```python
from build123d import *

# Parameters (mm, degrees)
SKETCH007_R     = 6
PAD006_DEPTH    = 30
POCKET_DEPTH    = 27
SKETCH009_W     = 9
SKETCH009_H     = 11
SKETCH009_H_2   = 3
POCKET001_DEPTH = 2


with BuildPart() as part:
    # Sketch007 → Pad006 (new body)
    with BuildSketch(Plane.XY):
        with BuildLine():
            ThreePointArc((83.613695, 29), (-88.5, 0), (83.613695, -29))
            Line((88.613695, -29), (83.613695, -29))
            Line((88.613695, 29), (88.613695, -29))
            Line((83.613695, 29), (88.613695, 29))
        make_face()
        with Locations((43.046276, 63.61895)):
            Circle(SKETCH007_R, mode=Mode.SUBTRACT)
        with Locations((54.046276, 52)):
            Circle(SKETCH007_R, mode=Mode.SUBTRACT)
        with Locations((65.046276, 40.38105)):
            Circle(SKETCH007_R, mode=Mode.SUBTRACT)
    extrude(amount=-PAD006_DEPTH)

    # Sketch008 → Pocket (cut)
    with BuildSketch(Plane.XY):
        with BuildLine():
            ThreePointArc((83.230103, 27), (-87.5, 0), (83.230103, -27))
            Line((83.230103, -27), (87.230103, -27))
            Line((87.230103, -27), (87.230103, 27))
            Line((87.230103, 27), (83.230103, 27))
        make_face()
    extrude(amount=-POCKET_DEPTH, mode=Mode.SUBTRACT)

    # Sketch009 (on Face6 of Pocket) → Pocket001 (cut)
    with BuildSketch(Plane.YZ.offset(88.613695)):
        with Locations((18, -19.5)):
            Rectangle(SKETCH009_W, SKETCH009_H)
        with Locations((-13.5, -23.5)):
            Rectangle(SKETCH009_W, SKETCH009_H_2)
    extrude(amount=-POCKET001_DEPTH, mode=Mode.SUBTRACT)


solid = part.part
```
CAD build for the part. Positions are in the model's coordinates, mm. A direction names the side the tool comes from. Coordinates: 2 decimals unless noted, no trailing zeros. Loops run counter-clockwise (first coordinate to the right, second up) from the corner with the lowest first, then second, coordinate; pieces in that order, holes last. Notation, with made-up numbers: (38.5, 88) - (89.5, 88) arc R28 ccw to (89.5, 125) - close; hole circle Ø10 at (-24.75, 43). An arc over 180 degrees is marked (long way). Return JSON: item names as keys, results as strings.
1. Mould opens along X. For faces 1 (the cylindrical face through (46.27, 68.68, -28.48)), 2 (the flat face through (85, -27, -13)), 3 (the flat face through (86, 29, -15)), 4 (the cylindrical face through (-88.43, 3.48, -14.79)) say: released by +X, released by -X, zero draft, split by the parting line, or undercut.
Result:
{"face 1": "undercut", "face 2": "undercut", "face 3": "zero draft", "face 4": "split by the parting line"}
2. Band-saw the part on D-D (x = 0). Give the cut face in (y, z), and give its area (3 significant figures).
Result:
{"outline": "(-88.5, -30) - (88.5, -30) - (88.5, 0) - (87.5, 0) - (87.5, -27) - (-87.5, -27) - (-87.5, 0) - (-88.5, 0) - close", "area": "585 mm2"}
3. Band-saw the part on A-A (z = -11.75). Give the cut face in (x, y).
Result:
{"outline": "(83.61, -29) - (88.61, -29) - (88.61, 29) - (83.61, 29) arc R88.5 ccw (long way) to start; hole (83.23, -27) - (87.23, -27) - (87.23, 27) - (83.23, 27) arc R87.5 ccw (long way) to start"}
4. Band-saw the part on B-B (x = 43). Give the cut face in (y, z).
Result:
{"outline": "(-77.35, -30) - (57.62, -30) - (57.62, -27) - (-76.21, -27) - (-76.21, 0) - (-77.35, 0) - close; (69.62, -30) - (77.35, -30) - (77.35, 0) - (76.21, 0) - (76.21, -27) - (69.62, -27) - close"}
5. Band-saw the part on C-C (y = -13.5). Give the cut face in (x, z), and give its area (3 significant figures).
Result:
{"outline": "(-87.46, -30) - (88.61, -30) - (88.61, -25) - (87.23, -25) - (87.23, -27) - (-86.45, -27) - (-86.45, 0) - (-87.46, 0) - close; (87.23, -22) - (88.61, -22) - (88.61, 0) - (87.23, 0) - close", "area": "589 mm2"}
6. Probe L1, parallel to Y at x = 0, z = -19.75; L2, parallel to Z at x = -25.5, y = -29; L3, parallel to X at y = 36.5, z = -4.5. List the from-to ranges inside material, lowest first. Write a range as from..to.
Result:
{"L1": "y = -88.5..-87.5, 87.5..88.5", "L2": "z = -30..-27", "L3": "x = -80.62..-79.52, 79.52..80.62"}
7. 3-axis set-ups, long thin cutter, end or side, ignore diameter. For faces 5 (the flat face through (86, -29, -15)), 6 (the cylindrical face through (60.285, 36.73, -28.479)), 7 (the flat face through (-1, 1, -27)): which of +Z, -Z, +X, -X, +Y, -Y reach the whole face in a straight line?
Result:
{"face 5": "+Z, -Z, +X, -Y", "face 6": "+Z, -Z", "face 7": "+Z"}
8. Drop flat-ended pins along their axis: pin 1 (10 mm diameter, centred on y = 13.5, z = -14, fed in from -X); pin 2 (10 mm diameter, centred on x = -2, y = 7, fed in from +Z); pin 3 (6 mm diameter, centred on x = 1, z = -4, fed in from -Y). Give the stop position or say it passes through.
Result:
{"pin 1": "stops at x = -88.09", "pin 2": "stops at z = -27", "pin 3": "stops at y = -88.5"}
